```python
from build123d import *

# Parameters (mm, degrees)
SKETCH1_R                    = 2.0828
BOSS_EXTRUDE1_DEPTH          = 3.175
F_18_0_1695_DIAMETER_HOLE1_D = 4.3053
CUT_EXTRUDE2_DEPTH           = 3.175
MIRROR1_COPY_1_DEPTH         = 3.175


with BuildPart() as part:
    # Sketch1 → Boss-Extrude1 (new body)
    with BuildSketch(Plane(origin=(0, 0, 0), x_dir=(1, 0, 0), z_dir=(0, 1, 0))):
        with BuildLine():
            Line((0, 0), (0, 49.391408666))
            ThreePointArc((0, 49.391408666), (0.383256806, 51.318170741), (1.474679849, 52.951600757))
            Line((1.474679849, 52.951600757), (10.45493597, 61.931856878))
            ThreePointArc((10.45493597, 61.931856878), (15.941890136, 63.023279921), (19.05, 58.371664787))
            Line((19.05, 58.371664787), (19.05, 0))
            Line((19.05, 0), (0, 0))
        make_face()
        with Locations(Location((14.015128061, 58.371664787, 0), (0, 0, 270))):
            Circle(SKETCH1_R, mode=Mode.SUBTRACT)
        with Locations(Location((5.034871939, 49.391408666, 0), (0, 0, 270))):
            Circle(SKETCH1_R, mode=Mode.SUBTRACT)
        with BuildLine():
            Line((13.164967985, 49.439274202), (3.639967985, 39.914274202))
            ThreePointArc((3.639967985, 39.914274202), (3.295841242, 38.184232238), (4.7625, 37.204242187))
            Line((4.7625, 37.204242187), (14.2875, 37.204242187))
            ThreePointArc((14.2875, 37.204242187), (15.410032015, 37.669210172), (15.875, 38.791742187))
            Line((15.875, 38.791742187), (15.875, 48.316742187))
            ThreePointArc((15.875, 48.316742187), (14.895009949, 49.783400945), (13.164967985, 49.439274202))
        make_face(mode=Mode.SUBTRACT)
    boss_extrude1 = extrude(amount=BOSS_EXTRUDE1_DEPTH)

    # #18 (0.1695) Diameter Hole1 (through all)
    with Locations(Plane(origin=(0, 0, 0), x_dir=(-1, 0, 0), z_dir=(0, -1, 0))):
        with Locations((-14.015128061, 58.371664787), (-5.034871939, 49.391408666)):
            f_18_0_1695_diameter_hole1 = Hole(F_18_0_1695_DIAMETER_HOLE1_D / 2)

    # Sketch5 → Cut-Extrude2 (cut)
    with BuildSketch(Plane(origin=(0, 3.175, 0), x_dir=(1, 0, 0), z_dir=(0, 1, 0))):
        with BuildLine():
            Line((14.2875, 34.664242187), (4.7625, 34.664242187))
            ThreePointArc((4.7625, 34.664242187), (3.639967985, 34.199274202), (3.175, 33.076742187))
            Line((3.175, 33.076742187), (3.175, 27.577480873))
            ThreePointArc((3.175, 27.577480873), (3.96875, 26.202665545), (5.55625, 26.202665545))
            Line((5.55625, 26.202665545), (15.08125, 31.701926859))
            ThreePointArc((15.08125, 31.701926859), (15.820907249, 33.487617421), (14.2875, 34.664242187))
        make_face()
        with BuildLine():
            Line((13.49375, 27.852443939), (3.96875, 22.353182625))
            ThreePointArc((3.96875, 22.353182625), (3.229092751, 20.567492062), (4.7625, 19.390867296))
            Line((4.7625, 19.390867296), (14.2875, 19.390867296))
            ThreePointArc((14.2875, 19.390867296), (15.410032015, 19.855835281), (15.875, 20.978367296))
            Line((15.875, 20.978367296), (15.875, 26.47762861))
            ThreePointArc((15.875, 26.47762861), (15.08125, 27.852443939), (13.49375, 27.852443939))
        make_face()
    cut_extrude2 = extrude(amount=-CUT_EXTRUDE2_DEPTH, mode=Mode.SUBTRACT)

    # Mirror2: Cut-Extrude2 across plane
    add(cut_extrude2.mirror(Plane(origin=(0, 0, -18.120867296), x_dir=(1, 0, 0), z_dir=(0, 0, -1))), mode=Mode.SUBTRACT)

    # Mirror1: Boss-Extrude1, #18 (0.1695) Diameter Hole1, Cut-Extrude2 across plane
    add(boss_extrude1.mirror(Plane(origin=(19.05, 3.175, 0), x_dir=(1, 0, 0), z_dir=(0, 0, -1))))
    add(f_18_0_1695_diameter_hole1.mirror(Plane(origin=(19.05, 3.175, 0), x_dir=(1, 0, 0), z_dir=(0, 0, -1))), mode=Mode.SUBTRACT)
    add(cut_extrude2.mirror(Plane(origin=(19.05, 3.175, 0), x_dir=(1, 0, 0), z_dir=(0, 0, -1))), mode=Mode.SUBTRACT)

    # Mirror1 copy 1 sketch → Mirror1 copy 1 (cut)
    with BuildSketch(Plane(origin=(0, 3.175, 36.241734593), x_dir=(1, 0, 0), z_dir=(0, 1, 0))):
        with BuildLine():
            Line((14.2875, 34.664242187), (4.7625, 34.664242187))
            ThreePointArc((4.7625, 34.664242187), (3.639967985, 34.199274202), (3.175, 33.076742187))
            Line((3.175, 33.076742187), (3.175, 27.577480873))
            ThreePointArc((3.175, 27.577480873), (3.96875, 26.202665545), (5.55625, 26.202665545))
            Line((5.55625, 26.202665545), (15.08125, 31.701926859))
            ThreePointArc((15.08125, 31.701926859), (15.820907249, 33.487617421), (14.2875, 34.664242187))
        make_face()
        with BuildLine():
            Line((13.49375, 27.852443939), (3.96875, 22.353182625))
            ThreePointArc((3.96875, 22.353182625), (3.229092751, 20.567492062), (4.7625, 19.390867296))
            Line((4.7625, 19.390867296), (14.2875, 19.390867296))
            ThreePointArc((14.2875, 19.390867296), (15.410032015, 19.855835281), (15.875, 20.978367296))
            Line((15.875, 20.978367296), (15.875, 26.47762861))
            ThreePointArc((15.875, 26.47762861), (15.08125, 27.852443939), (13.49375, 27.852443939))
        make_face()
    extrude(amount=-MIRROR1_COPY_1_DEPTH, mode=Mode.SUBTRACT)


solid = part.part
```
CAD build for the part. Positions are in the model's coordinates, mm. A direction names the side the tool comes from. Give positions to 0.01 mm unless a question says otherwise; leave off trailing zeros. Write each loop counter-clockwise with the first axis right and the second up, starting at its lowest first coordinate (ties: lowest second). Pieces come first, ordered by that corner, then holes. Notation, with made-up numbers: M -20.5,-35.75 L 31.5,-35.75 A17 ccw 31.5,-23.75 Z; hole C -29,81.25 d3. An arc over 180 degrees is marked long. Return JSON: item names as keys, results as strings. Group by question number.
(1) Flat gauge pins, fed straight in: pin 1 Ø5.5 at (x, z) = (5.03, -49.39) entering from +Y (3 decimals); pin 2 Ø1.5 at (x, y) = (8.5, 2.5) entering from +Z. Where does each tip first touch, or does it go through?
(2) Drill centre lines: L1, parallel to X at y = 0.85, z = 9.5; L2, parallel to X at y = 1.65, z = -34.5; L3, parallel to X at y = 2.65, z = -2.5. Where is each one in solid material? Low to high. Write a range as [from, to].
(3) 3-axis set-ups, long thin cutter, end or side, ignore diameter. For faces 4 (the face through (15.1, 1.6, 8.4)), 5 (the face through (5.902, 1.565, -57.379)): which of +Z, -Z, +X, -X, +Y, -Y reach the whole face in a straight line?
(4) Band-saw the part on A-A (z = 30.5). Give the cut face in (x, y) (3 decimals), and give its area (3 significant figures).
(5) Mould opens along Z. For faces 1 (the face through (0.37, 1.57, -51.29)), 2 (the face through (15.1, 1.6, -8.4)), 3 (the face through (4.57, 1.61, 47.29)) say: pulls with the +Z half, pulls with the -Z half, needs draft (parallel to the pull), parting line crosses it, or undercut.
(6) Band-saw the part on C-C (z = -30). Give the cut face in (x, y) (3 decimals), and give its area (3 significant figures).
(7) Band-saw the part on D-D (x = 17.75). Give the cut face in (y, z) (3 decimals), and give its area (3 significant figures).
(8) Band-saw the part on B-B (y = 1.65). State how many separate pieces and enclosed holes the cut face has, and give its area (3 significant figures).
Entries:
{
 "1": {"pin 1": "stops at y = 3.175", "pin 2": "stops at z = 60.73"},
 "2": {"L1": "x = [0, 3.41], [6.49, 11.57], [15.85, 19.05]", "L2": "x = [0, 4.06], [14.99, 19.05]", "L3": "x = [0, 3.32], [15.73, 19.05]"},
 "3": {"face 4": "+Y, -Y", "face 5": "-Z, -X, +Y, -Y"},
 "4": {"outline": "M 0,0 L 3.175,0 L 3.175,3.175 L 0,3.175 Z; M 12.999,0 L 19.05,0 L 19.05,3.175 L 12.999,3.175 Z", "area": "29.3 mm^2"},
 "5": {"face 1": "pulls with the -Z half", "face 2": "undercut", "face 3": "undercut"},
 "6": {"outline": "M 0,0 L 3.175,0 L 3.175,3.175 L 0,3.175 Z; M 12.133,0 L 19.05,0 L 19.05,3.175 L 12.133,3.175 Z", "area": "32.0 mm^2"},
 "7": {"outline": "M 0,-61.748 L 3.175,-61.748 L 3.175,61.748 L 0,61.748 Z", "area": "392 mm^2"},
 "8": {"separate pieces": "1", "enclosed holes": "14", "area": "1,390 mm^2"}
}
